The listing builds one solid part. Answer for the finished solid, in the listing's coordinates (mm). A direction names the side the tool comes from. Give positions to 0.01 mm unless a question says otherwise; leave off trailing zeros. Loops run counter-clockwise (first coordinate to the right, second up) from the corner with the lowest first, then second, coordinate; pieces in that order, holes last. Notation, with made-up numbers: (72, -28.5) - (108, -28.5) arc R5 ccw to (108, -21.5) - close; hole circle Ø9 at (74.5, 73.5). An arc over 180 degrees is marked (long way). Write item = value, one per line. Start each with the question number.
1) The part is cut by section A-A on y = -14. Write down the section's boundary in (x, z) (3 decimals), plus the area to 3 significant figures.
2) Which of the six approach directions +Z, -Z, +X, -X, +Y, -Y give full straight-line access (tool end or side, diameter ignored) to faces 5 (the flat face through (-10, 0, 6.35)), 6 (the flat face through (62.031, 0, 5)), 7 (the flat face through (-80.169, 0, 5))?
3) Consider probe 1 along X at (y, z) = (1.5, 5); probe 2 along X at (y, z) = (-13.5, 4); probe 3 along X at (y, z) = (-9.5, 2.25). Determine where each line is inside the solid, lowest interval first.
4) Flat-ended cylindrical pins translate along their axes: P1, Ø2.5, axis at x = -83.28, y = 9.21, coming from the -Z side; P2, Ø1.6, axis at y = -6, z = 5, coming from the +X side; P3, Ø3, axis at x = -82, y = 1.5, coming from the +Z side (3 decimals); P4, Ø1.6, axis at y = 9, z = 4.5, coming from the -X side. Find the tip coordinate at first contact, or state that the pin passes through.
5) The mould has two halves that part along Y. Classify faces 1 (the cylindrical face through (-2.9, -1.62, 3.22)), 2 (the flat face through (77.58, 8.94, 3.22)), 3 (the flat face through (77.32, -9.2, 3.22)), 4 (the flat face through (68.381, 0, 5)): +Y half, -Y half, draft (parallel to the pull), parting line (faces both ways), or undercut.
from build123d import *

# Parameters (mm, degrees)
SKETCH1_W                                         = 173.0375
SKETCH1_H                                         = 36.27882
EXTRUDE2_DEPTH                                    = 6.35
SKETCH8_W                                         = 6.35
SKETCH8_H                                         = 36.27882
EXTRUDE7_DEPTH                                    = 3.175
CSK_FOR_3_FLAT_HEAD_SOCKET_CAP_SCREW1_D           = 2.794
CSK_FOR_3_FLAT_HEAD_SOCKET_CAP_SCREW1_CSINK_D     = 5.51688
CSK_FOR_3_FLAT_HEAD_SOCKET_CAP_SCREW1_CSINK_ANGLE = 82
CSK_FOR_3_FLAT_HEAD_SOCKET_CAP_SCREW2_D           = 2.794
CSK_FOR_3_FLAT_HEAD_SOCKET_CAP_SCREW2_CSINK_D     = 5.51688
CSK_FOR_3_FLAT_HEAD_SOCKET_CAP_SCREW2_CSINK_ANGLE = 82
CSK_FOR_3_FLAT_HEAD_SOCKET_CAP_SCREW3_D           = 2.794
CSK_FOR_3_FLAT_HEAD_SOCKET_CAP_SCREW3_CSINK_D     = 5.51688
CSK_FOR_3_FLAT_HEAD_SOCKET_CAP_SCREW3_CSINK_ANGLE = 82
EXTRUDE8_DEPTH                                    = 89.627618702
SKETCH19_R                                        = 2.656568676
EXTRUDE9_DEPTH                                    = 89.627618702


with BuildPart() as part:
    # Sketch1 → Extrude2 (new body)
    with BuildSketch(Plane.XY):
        Rectangle(SKETCH1_W, SKETCH1_H)
    extrude(amount=EXTRUDE2_DEPTH)

    # Sketch8 → Extrude7 (cut)
    with BuildSketch(Plane.XY.offset(6.35)):
        with Locations((-83.34375, 0)):
            Rectangle(SKETCH8_W, SKETCH8_H)
        with Locations((65.20561, 0)):
            Rectangle(SKETCH8_W, SKETCH8_H)
    extrude(amount=-EXTRUDE7_DEPTH, mode=Mode.SUBTRACT)

    # CSK for #3 Flat Head Socket Cap Screw1 (through all)
    with Locations(Plane(origin=(-27.747731188, -5.395978674, 0), x_dir=(-1, 0, 0), z_dir=(0, 0, -1))):
        with Locations((55.533788812, -4.331019161)):
            CounterSinkHole(CSK_FOR_3_FLAT_HEAD_SOCKET_CAP_SCREW1_D / 2, CSK_FOR_3_FLAT_HEAD_SOCKET_CAP_SCREW1_CSINK_D / 2, counter_sink_angle=CSK_FOR_3_FLAT_HEAD_SOCKET_CAP_SCREW1_CSINK_ANGLE)

    # CSK for #3 Flat Head Socket Cap Screw2 (through all)
    with Locations(Plane(origin=(-27.747731188, -5.395978674, 0), x_dir=(-1, 0, 0), z_dir=(0, 0, -1))):
        with Locations((55.533788812, 14.608526561)):
            CounterSinkHole(CSK_FOR_3_FLAT_HEAD_SOCKET_CAP_SCREW2_D / 2, CSK_FOR_3_FLAT_HEAD_SOCKET_CAP_SCREW2_CSINK_D / 2, counter_sink_angle=CSK_FOR_3_FLAT_HEAD_SOCKET_CAP_SCREW2_CSINK_ANGLE)

    # CSK for #3 Flat Head Socket Cap Screw3 (through all)
    with Locations(Plane(origin=(-27.747731188, -5.395978674, 0), x_dir=(-1, 0, 0), z_dir=(0, 0, -1))):
        with Locations((-91.600791188, -4.318251326), (-91.600791188, 15.110208674)):
            CounterSinkHole(CSK_FOR_3_FLAT_HEAD_SOCKET_CAP_SCREW3_D / 2, CSK_FOR_3_FLAT_HEAD_SOCKET_CAP_SCREW3_CSINK_D / 2, counter_sink_angle=CSK_FOR_3_FLAT_HEAD_SOCKET_CAP_SCREW3_CSINK_ANGLE)

    # Sketch18 → Extrude8 (cut, through all)
    with BuildSketch(Plane.XY.offset(6.35)):
        Polygon((86.51875, 0), (68.38061, 18.13941), (113.519162523, 18.13941), (113.519162523, -18.13941), (68.38061, -18.13941), align=None)
    extrude(amount=-EXTRUDE8_DEPTH, mode=Mode.SUBTRACT)

    # Sketch19 → Extrude9 (cut, through all)
    with BuildSketch(Plane.XY.offset(6.35)):
        with Locations((-0.79375, 0)):
            Circle(SKETCH19_R)
    extrude(amount=-EXTRUDE9_DEPTH, mode=Mode.SUBTRACT)


solid = part.part
Answer below:
q1.outline = (-86.519, 0) - (72.52, 0) - (72.52, 6.35) - (68.381, 6.35) - (68.381, 3.175) - (62.031, 3.175) - (62.031, 6.35) - (-80.169, 6.35) - (-80.169, 3.175) - (-86.519, 3.175) - close
q1.area = 970 mm2
q2.face_5 = +Z, +X, -X, +Y, -Y
q2.face_6 = +Z, +Y, -Y
q2.face_7 = +Z, -X, +Y, -Y
q3.probe_1 = -80.17 to -2.99, 1.4 to 62.03, 68.38 to 85.02
q3.probe_2 = -80.17 to 62.03, 68.38 to 73.02
q3.probe_3 = -86.52 to -84.66, -81.9 to 62.47, 65.23 to 77.02
q4.P1 = through
q4.P2 = 81.32
q4.P3 = 3.175
q4.P4 = -80.17
q5.face_1 = undercut
q5.face_2 = +Y half
q5.face_3 = -Y half
q5.face_4 = draft
